from build123d import *

# Parameters (mm, degrees)
SKETCH2_R           = 3.15
BOSS_EXTRUDE1_DEPTH = 2


with BuildPart() as part:
    # Sketch2 → Boss-Extrude1 (new body)
    with BuildSketch(Plane(origin=(0, 0, 0), x_dir=(1, 0, 0), z_dir=(0, 1, 0))):
        with BuildLine():
            Line((0.553571832, -40.497268471), (11.553571832, -40.497268471))
            ThreePointArc((11.553571832, -40.497268471), (14.735552347, -39.179248986), (16.053571832, -35.997268471))
            Line((16.053571832, -35.997268471), (16.053571832, -22.997268471))
            ThreePointArc((16.053571832, -22.997268471), (14.735552347, -19.815287955), (11.553571832, -18.497268471))
            Line((11.553571832, -18.497268471), (0.553571832, -18.497268471))
            ThreePointArc((0.553571832, -18.497268471), (-2.628408684, -19.815287955), (-3.946428168, -22.997268471))
            Line((-3.946428168, -22.997268471), (-3.946428168, -35.997268471))
            ThreePointArc((-3.946428168, -35.997268471), (-2.628408684, -39.179248986), (0.553571832, -40.497268471))
        make_face()
        with Locations(Location((11.553571832, -35.997268471, 0), (0, 0, 270))):
            Circle(SKETCH2_R, mode=Mode.SUBTRACT)
        with Locations(Location((11.553571832, -22.997268471, 0), (0, 0, 90))):
            Circle(SKETCH2_R, mode=Mode.SUBTRACT)
        with Locations(Location((0.553571832, -22.997268471, 0), (0, 0, 270))):
            Circle(SKETCH2_R, mode=Mode.SUBTRACT)
        with Locations(Location((0.553571832, -35.997268471, 0), (0, 0, 90))):
            Circle(SKETCH2_R, mode=Mode.SUBTRACT)
    extrude(amount=-BOSS_EXTRUDE1_DEPTH)


solid = part.part
Could you check a few things on this model? Use its own coordinates, in mm. Round coordinates to 2 decimals unless told otherwise and drop trailing zeros. Order: outer loops, then holes, each group sorted by start corner. A loop starts at its lowest first (then second) coordinate and runs counter-clockwise, first axis right, second up.
Q1. Imagine slicing it at C-C, the plane z = 22. List the corners of the cut face in (x, y) for me, then the cut area to 3 significant figures.
Geometry says:
outline: (-3.83, -2) - (-2.43, -2) - (-2.43, 0) - (-3.83, 0) - close; (3.54, -2) - (8.57, -2) - (8.57, 0) - (3.54, 0) - close; (14.54, -2) - (15.94, -2) - (15.94, 0) - (14.54, 0) - close
area: 15.6 mm2
Q2. Please list where these lines run through material, in increasing order: probe 1 along Z at (x, y) = (13.75, -1.8); probe 2 along X at (y, z) = (-1.25, 34); probe 3 along X at (y, z) = (-0.6, 23).
Geometry says:
probe 1: z = 19.07 to 20.74, 25.26 to 33.74, 38.26 to 39.92
probe 2: x = -3.95 to -1.88, 2.99 to 9.12, 13.99 to 16.05
probe 3: x = -3.95 to -2.6, 3.7 to 8.4, 14.7 to 16.05
Q3. I'm going to push a flat-ended pin straight in: P1, Ø7, axis at x = 11.55, z = 36, coming from the +Y side. Where does the tip first touch, or does it pass through?
Geometry says:
P1: stops at y = 0
Q4. Imagine slicing it at A-A, the plane y = -0.4. List the corners of the cut face in (x, z) for me.
Geometry says:
outline: (-3.95, 23) arc R4.5 ccw to (0.55, 18.5) - (11.55, 18.5) arc R4.5 ccw to (16.05, 23) - (16.05, 36) arc R4.5 ccw to (11.55, 40.5) - (0.55, 40.5) arc R4.5 ccw to (-3.95, 36) - close; hole circle Ø6.3 at (0.55, 23); hole circle Ø6.3 at (0.55, 36); hole circle Ø6.3 at (11.55, 23); hole circle Ø6.3 at (11.55, 36)
Q5. Thinking about a two-plate mould opening in Z: for faces 1 (the face through (6, -1, 18.497)), 2 (the face through (13.47, -0.986, 25.497)), 3 (the face through (0.69, -0.99, 19.85)), 4 (the face through (6, -1, 40.497)), which applies, released by +Z, released by -Z, zero draft, split by the parting line, or undercut?
Geometry says:
face 1: released by -Z
face 2: undercut
face 3: undercut
face 4: released by +Z
Q6. Imagine slicing it at B-B, the plane x = -0.5. List the corners of the cut face in (y, z) for me, then the cut area to 3 significant figures.
Geometry says:
outline: (-2, 18.62) - (0, 18.62) - (0, 20.03) - (-2, 20.03) - close; (-2, 25.97) - (0, 25.97) - (0, 33.03) - (-2, 33.03) - close; (-2, 38.97) - (0, 38.97) - (0, 40.37) - (-2, 40.37) - close
area: 19.8 mm2
